Check sheet for the modelled part. Datum: model origin and axes. Units: mm. A direction names the side the tool comes from. Give positions to 0.01 mm unless a question says otherwise; leave off trailing zeros. Order: outer loops, then holes, each group sorted by start corner. A loop starts at its lowest first (then second) coordinate and runs counter-clockwise, first axis right, second up.
Item 1: Material ranges on line 1 along Y through (x, z) = (10, 0.9); line 2 along X through (y, z) = (10, 3.35); line 3 along Y through (x, z) = (10, 6.6), recorded low to high.
Item 2: Sectioned sample at D-D on x = 130. Record the boundary of the cut face in (y, z).
Item 3: Sectioned sample at C-C on y = 57. Record the boundary of the cut face in (x, z), and give its area (4 significant figures).
Item 4: Access from +Z, -Z, +X, -X, +Y, -Y to the whole of each face (thin tool, end or side, straight path). Record for faces 1 (the flat face through (140, 6, 4)), 2 (the flat face through (75, 26, 1)), 3 (the flat face through (117, 20, 4)), 4 (the flat face through (12, 8, 4.5)).
Item 5: Sectioned sample at A-A on x = 33.5. Record the boundary of the cut face in (y, z), and give its area (4 significant figures).
Item 6: Gauge pin test, flat ends, axial feed: P1, Ø9, axis at x = 80, y = 26, coming from the -Z side; P2, Ø3.5, axis at x = 40, y = 10, coming from the +Z side; P3, Ø0.8, axis at y = 27, z = 1, coming from the +X side. Record the tip position at first contact, or that the pin passes through.
Item 7: Sectioned sample at B-B on z = 7. Record the boundary of the cut face in (x, y), and give its area (3 significant figures).
Item 8: Release check for a two-part mould opening along Y. For faces 5 (the flat face through (71, 0, 4)), 6 (the flat face through (77, 23, 2.5)), 7 (the flat face through (95, 30, 4)) record: released by +Y, released by -Y, zero draft, split by the parting line, or undercut.
from build123d import *

# Parameters (mm, degrees)
PAD002_DEPTH      = 2.5
CYLINDER003_R     = 2.8
CYLINDER003_DEPTH = 15
CYLINDER004_R     = 1.5
CYLINDER004_DEPTH = 8.5
CYLINDER001_R     = 3.5
CYLINDER001_DEPTH = 4
CYLINDER_R        = 3.5
CYLINDER_DEPTH    = 4
CYLINDER002_R     = 3.5
CYLINDER002_DEPTH = 4
PAD001_DEPTH      = 2.5
PAD003_DEPTH      = 2.5
CYLINDER006_R     = 2.8
CYLINDER006_DEPTH = 15
CYLINDER005_R     = 1.5
CYLINDER005_DEPTH = 8.5
SKETCH_R          = 2
SKETCH_R_2        = 7
SKETCH_R_3        = 4
PAD_DEPTH         = 8.5


with BuildPart() as body002:
    # Sketch002 → Pad002 (new body)
    with BuildSketch(Plane.XY):
        Polygon((0, -3.2), (2.771281, -1.6), (2.771281, 1.6), (0, 3.2), (-2.771281, 1.6), (-2.771281, -1.6), align=None)
    extrude(amount=PAD002_DEPTH)


with BuildPart() as cylinder003:
    # Cylinder003 → Cylinder003 (new body)
    with BuildSketch(Plane.XY.offset(5.5)):
        Circle(CYLINDER003_R)
    extrude(amount=CYLINDER003_DEPTH)


with BuildPart() as fusion001:
    # Cylinder004 → Cylinder004 (new body)
    with BuildSketch(Plane.XY):
        Circle(CYLINDER004_R)
    extrude(amount=CYLINDER004_DEPTH)

    # Fusion001: union Body002, Cylinder003
    add(body002.part)
    add(cylinder003.part)


with BuildPart() as fusion001_1:
    # Fusion001 placement: moved
    add(fusion001.part.moved(Location((40, 10, 0))))


with BuildPart() as cylinder001:
    # Cylinder001 → Cylinder001 (new body)
    with BuildSketch(Plane(origin=(130, 10, 4.5), x_dir=(1, 0, 0), z_dir=(0, 0, 1))):
        Circle(CYLINDER001_R)
    extrude(amount=CYLINDER001_DEPTH)


with BuildPart() as cylinder:
    # Cylinder → Cylinder (new body)
    with BuildSketch(Plane(origin=(10, 10, 4.5), x_dir=(1, 0, 0), z_dir=(0, 0, 1))):
        Circle(CYLINDER_R)
    extrude(amount=CYLINDER_DEPTH)


with BuildPart() as cylinder002:
    # Cylinder002 → Cylinder002 (new body)
    with BuildSketch(Plane(origin=(10, 57, 4.5), x_dir=(1, 0, 0), z_dir=(0, 0, 1))):
        Circle(CYLINDER002_R)
    extrude(amount=CYLINDER002_DEPTH)


with BuildPart() as fusion:
    # Sketch001 → Pad001 (new body, symmetric)
    with BuildSketch(Plane.XY):
        Polygon((0, -5.773503), (5, -2.886751), (5, 2.886751), (0, 5.773503), (-5, 2.886751), (-5, -2.886751), align=None)
    extrude(amount=PAD001_DEPTH, both=True)


with BuildPart() as fusion_1:
    # Body001 placement: moved
    add(fusion.part.moved(Location((80, 26, 0))))

    # Fusion: union Cylinder001, Cylinder, Cylinder002
    add(cylinder001.part)
    add(cylinder.part)
    add(cylinder002.part)


with BuildPart() as body003:
    # Sketch003 → Pad003 (new body)
    with BuildSketch(Plane.XY):
        Polygon((0, -3.2), (2.771281, -1.6), (2.771281, 1.6), (0, 3.2), (-2.771281, 1.6), (-2.771281, -1.6), align=None)
    extrude(amount=PAD003_DEPTH)


with BuildPart() as cylinder006:
    # Cylinder006 → Cylinder006 (new body)
    with BuildSketch(Plane.XY.offset(5.5)):
        Circle(CYLINDER006_R)
    extrude(amount=CYLINDER006_DEPTH)


with BuildPart() as fusion003:
    # Cylinder005 → Cylinder005 (new body)
    with BuildSketch(Plane.XY):
        Circle(CYLINDER005_R)
    extrude(amount=CYLINDER005_DEPTH)

    # Fusion002: union Body003, Cylinder006
    add(body003.part)
    add(cylinder006.part)


with BuildPart() as fusion003_1:
    # Fusion002 placement: moved
    add(fusion003.part.moved(Location((90, 10, 0))))

    # Fusion003: union Fusion001, Fusion
    add(fusion001_1.part)
    add(fusion_1.part)


with BuildPart() as cut:
    # Sketch → Pad (new body)
    with BuildSketch(Plane.XY):
        with BuildLine():
            Line((0, 0), (0, 59))
            ThreePointArc((8, 67), (2.343146, 64.656854), (0, 59))
            Line((8, 67), (57, 67))
            ThreePointArc((65, 59), (62.656854, 64.656854), (57, 67))
            Line((65, 59), (65, 48))
            ThreePointArc((65, 48), (67.343146, 42.343146), (73, 40))
            Line((73, 40), (87, 40))
            ThreePointArc((95, 32), (92.656854, 37.656854), (87, 40))
            Line((95, 32), (95, 28))
            ThreePointArc((95, 28), (97.343146, 22.343146), (103, 20))
            Line((103, 20), (132, 20))
            ThreePointArc((140, 12), (137.656854, 17.656854), (132, 20))
            Line((140, 12), (140, 0))
            Line((140, 0), (0, 0))
        make_face()
        with Locations((10, 10)):
            Circle(SKETCH_R, mode=Mode.SUBTRACT)
        with Locations((10, 57)):
            Circle(SKETCH_R, mode=Mode.SUBTRACT)
        with Locations((33.5, 39)):
            Circle(SKETCH_R_2, mode=Mode.SUBTRACT)
        with Locations((80, 26)):
            Circle(SKETCH_R_3, mode=Mode.SUBTRACT)
        with Locations((130, 10)):
            Circle(SKETCH_R, mode=Mode.SUBTRACT)
    extrude(amount=PAD_DEPTH)

    # Cut: cut Fusion003
    add(fusion003_1.part, mode=Mode.SUBTRACT)


solid = cut.part
Report:
1. line 1: y = 0 to 8, 12 to 55, 59 to 67
1. line 2: x = 0 to 8, 12 to 38.5, 41.5 to 88.5, 91.5 to 128, 132 to 140
1. line 3: y = 0 to 6.5, 13.5 to 53.5, 60.5 to 67
2. outline: (0, 0) - (8, 0) - (8, 4.5) - (6.5, 4.5) - (6.5, 8.5) - (0, 8.5) - close; (12, 0) - (20, 0) - (20, 8.5) - (13.5, 8.5) - (13.5, 4.5) - (12, 4.5) - close
3. outline: (0, 0) - (8, 0) - (8, 4.5) - (6.5, 4.5) - (6.5, 8.5) - (0, 8.5) - close; (12, 0) - (65, 0) - (65, 8.5) - (13.5, 8.5) - (13.5, 4.5) - (12, 4.5) - close
3. area: 506.5 mm2
4. face 1: +Z, -Z, +X, +Y, -Y
4. face 2: -Z
4. face 3: +Z, -Z, +X, +Y
4. face 4: +Z
5. outline: (0, 0) - (32, 0) - (32, 8.5) - (0, 8.5) - close; (46, 0) - (67, 0) - (67, 8.5) - (46, 8.5) - close
5. area: 450.5 mm2
6. P1: stops at z = 2.5
6. P2: stops at z = 5.5
6. P3: stops at x = 95.12
7. outline: (0, 0) - (140, 0) - (140, 12) arc R8 ccw to (132, 20) - (103, 20) arc R8 cw to (95, 28) - (95, 32) arc R8 ccw to (87, 40) - (73, 40) arc R8 cw to (65, 48) - (65, 59) arc R8 ccw to (57, 67) - (8, 67) arc R8 ccw to (0, 59) - close; hole circle Ø7 at (10, 10); hole circle Ø7 at (10, 57); hole circle Ø14 at (33.5, 39); hole circle Ø5.6 at (40, 10); hole circle Ø8 at (80, 26); hole circle Ø5.6 at (90, 10); hole circle Ø7 at (130, 10)
7. area: 6,060 mm2
8. face 5: released by -Y
8. face 6: undercut
8. face 7: zero draft
